from build123d import *

# Parameters (mm, degrees)
F0_W     = 50
F0_H     = 150
F1_DEPTH = 100
F2_R     = 30
F3_DEPTH = 40
F4_R     = 35
F5_R     = 35


with BuildPart() as f1:
    # F0 (on Top) → F1 (new body)
    with BuildSketch(Plane.XY):
        with Locations((-151.100701, 43.27358)):
            Rectangle(F0_W, F0_H)
    extrude(amount=F1_DEPTH)

    # F2 (on face) → F3 (join)
    with BuildSketch(Plane(origin=(-176.100701, 0, 0), x_dir=(0, -1, 0), z_dir=(-1, 0, 0))):
        with Locations((-12.505785, 54.520387)):
            Circle(F2_R)
    extrude(amount=F3_DEPTH)

    # F4
    f4_edges = [f1.edges().sort_by_distance(p)[0] for p in [
        (-151.100701, 118.27358, 100),
    ]]
    fillet(f4_edges, radius=F4_R)

    # F5
    f5_edges = [f1.edges().sort_by_distance(p)[0] for p in [
        (-151.100701, -31.72642, 100),
    ]]
    fillet(f5_edges, radius=F5_R)


solid = f1.part
Could you check a few things on this model? Use its own coordinates, in mm. A direction names the side the tool comes from. Coordinates: 2 decimals unless noted, no trailing zeros. Write each loop counter-clockwise with the first axis right and the second up, starting at its lowest first coordinate (ties: lowest second). Pieces come first, ordered by that corner, then holes. Notation, with made-up numbers: (-9, 61.25) - (18, 61.25) arc R30 ccw to (18, 90.25) - close; hole circle Ø7 at (2, 1). An arc over 180 degrees is marked (long way). Write item = value, one per line.
1) Suppose I cut it at C-C on y = 20.5. Please give me the cut outline in (x, z).
Result set:
outline = (-216.1, 25.61) - (-176.1, 25.61) - (-176.1, 0) - (-126.1, 0) - (-126.1, 100) - (-176.1, 100) - (-176.1, 83.44) - (-216.1, 83.44) - close
2) Will these pins go through, and if not, where does the flat tip stop? pin 1 Ø10 at (x, z) = (-151, 89) entering from +Y; pin 2 Ø10 at (x, y) = (-155.5, 64.5) entering from -Z.
Result set:
pin_1 = 112.67
pin_2 = 0
3) Suppose I cut it at D-D on y = 53. Please give me the cut outline in (x, z).
Result set:
outline = (-176.1, 0) - (-126.1, 0) - (-126.1, 100) - (-176.1, 100) - close
4) Please list where these lines run through material, in increasing order: line 1 (Z direction, x = -143, y = 2); line 2 (Y direction, x = -193, z = 55.5); line 3 (X direction, y = 77, z = 10.5). Write a range as [from, to].
Result set:
line_1 = [0, 99.98]
line_2 = [-17.48, 42.49]
line_3 = [-176.1, -126.1]
5) For faces 1 (the cylindrical face through (-195.821, -1.337, 27.905)), 2 (the flat face through (-151, 44, 100)), which set-ups out of +Z, -Z, +X, -X, +Y, -Y let a thin tool reach every point of the face, with its end or its side?
Result set:
face_1 = -X
face_2 = +Z, +X, -X, +Y, -Y
6) Suppose I cut it at B-B on z = 69. Please give me the cut outline in (x, y), plus the area to 3 significant figures.
Result set:
outline = (-216.1, -13.77) - (-176.1, -13.77) - (-176.1, -31.5) - (-126.1, -31.5) - (-126.1, 118.04) - (-176.1, 118.04) - (-176.1, 38.78) - (-216.1, 38.78) - close
area = 9,580 mm2
7) Suppose I cut it at A-A on x = -174. Please give me the cut outline in (y, z), plus the area to 3 significant figures.
Result set:
outline = (-31.73, 0) - (118.27, 0) - (118.27, 65) arc R35 ccw to (83.27, 100) - (3.27, 100) arc R35 ccw to (-31.73, 65) - close
area = 14,500 mm2
